Geometry check sheet. Reference: the model listing, model coordinates, mm. A direction names the side the tool comes from. Coordinates: 2 decimals unless noted, no trailing zeros. Write each loop counter-clockwise with the first axis right and the second up, starting at its lowest first coordinate (ties: lowest second). Pieces come first, ordered by that corner, then holes. Notation, with made-up numbers: (-27, -15) -> (28, -15) arc R27 ccw to (28, 12) -> close; hole circle Ø6 at (78, -32). An arc over 180 degrees is marked (long way). Answer in a Markdown table with one row per item. Add a question column.
1. Cross-section at D-D on z = -6.5. Record the cut outline in (x, y) (3 decimals), and give its area (3 significant figures).
2. Cross-section at C-C on x = 10. Record the cut outline in (y, z) (3 decimals).
3. Set-up check for faces 3 (the flat face through (0, -30, 3.35)), 4 (the flat face through (0, -61.675, 4)): record each of +Z, -Z, +X, -X, +Y, -Y from which the full face is reachable in a straight line by a thin tool's end or side.
4. Mould release check, pull along X, two halves, no side actions. Record for faces 1 (the cylindrical face through (-8.946, -31.269, -0.672)), 2 (the flat face through (0, 0, 4)): pulls with the +X half, pulls with the -X half, needs draft (parallel to the pull), parting line crosses it, or undercut.
5. Scan lines: L1, parallel to X at y = -46.5, z = -10; L2, parallel to Z at x = -1, y = -56.5; L3, parallel to Z at x = -9.5, y = -56. Record each from-to range of solid material in increasing order. Write a range as from..to.
6. Cross-section at B-B on y = -19. Record the cut outline in (x, z).
7. Depth check by flat-ended pin: P1, Ø5.5, axis at y = -43, z = -1.5, coming from the +X side; P2, Ø12, axis at y = -23, z = -12.5, coming from the -X side; P3, Ø1, axis at x = 6, y = -16.5, coming from the +Z side; P4, Ø3, axis at y = -16.5, z = -5, coming from the -X side. Enter the tip coordinate at first touch or a pass-through.
8. Cross-section at A-A on z = 10. Record the cut outline in (x, y) (3 decimals).
```python
from build123d import *

# Parameters (mm, degrees)
SKETCH1_W                   = 6.7
SKETCH1_H                   = 6.7
BOSS_EXTRUDE1_DEPTH         = 61.675
TAP_DRILL_FOR_M3X0_5_TAP1_D = 2.5


with BuildPart() as part:
    # Sketch1 → Boss-Extrude1 (new body)
    # profile 1 of 2: a face of its own
    with BuildSketch(Plane(origin=(0, 0, 0), x_dir=(1, 0, 0), z_dir=(0, 1, 0))):
        with BuildLine():
            ThreePointArc((0, -17.5), (12.374368671, -12.374368671), (17.5, 0))
            ThreePointArc((17.5, 0), (7.362522242, -7.362522242), (0, -17.5))
        make_face()
    # profile 2 of 2: a face of its own
    with BuildSketch(Plane(origin=(0, 0, 0), x_dir=(1, 0, 0), z_dir=(0, 1, 0))):
        with BuildLine():
            ThreePointArc((0, -17.5), (7.362522242, -7.362522242), (17.5, 0))
            ThreePointArc((17.5, 0), (-12.374368671, 12.374368671), (0, -17.5))
        make_face()
        Rectangle(SKETCH1_W, SKETCH1_H, mode=Mode.SUBTRACT)
    extrude(amount=-BOSS_EXTRUDE1_DEPTH)

    # Tap Drill for M3x0.5 Tap1 (through all)
    with Locations(Plane(origin=(0, 0, -10), x_dir=(0, 0, 1), z_dir=(0, 1, 0))):
        with Locations((0, 0), (10, 10), (10, -10), (20, 0)):
            Hole(TAP_DRILL_FOR_M3X0_5_TAP1_D / 2)


solid = part.part
```
Results found:
| question | item | result |
|---|---|---|
| 1 | outline | (-16.248, -61.675) -> (16.248, -61.675) -> (16.248, 0) -> (-16.248, 0) -> close |
| 1 | area | 2,000 mm^2 |
| 2 | outline | (-61.675, -14.361) -> (0, -14.361) -> (0, -1.25) -> (-61.675, -1.25) -> close; (-61.675, 1.25) -> (0, 1.25) -> (0, 14.361) -> (-61.675, 14.361) -> close |
| 3 | face 3 | +Y, -Y |
| 3 | face 4 | +Z, -Z, +X, -X, -Y |
| 4 | face 1 | undercut |
| 4 | face 2 | needs draft |
| 5 | L1 | x = -14.36..-1.25, 1.25..14.36 |
| 5 | L2 | z = -17.47..-10.75, -9.25..-3.35, 3.35..9.25, 10.75..17.47 |
| 5 | L3 | z = -14.7..-1.15, 1.15..14.7 |
| 6 | outline | circle Ø35 at (0, 0); hole circle Ø2.5 at (-10, 0); hole (-3.35, -3.35) -> (3.35, -3.35) -> (3.35, 3.35) -> (-3.35, 3.35) -> close; hole circle Ø2.5 at (0, -10); hole circle Ø2.5 at (0, 10); hole circle Ø2.5 at (10, 0) |
| 7 | P1 | stops at x = 17.5 |
| 7 | P2 | stops at x = -16.25 |
| 7 | P3 | stops at z = 16.61 |
| 7 | P4 | stops at x = -17.15 |
| 8 | outline | (-14.361, -61.675) -> (-1.25, -61.675) -> (-1.25, 0) -> (-14.361, 0) -> close; (1.25, -61.675) -> (14.361, -61.675) -> (14.361, 0) -> (1.25, 0) -> close |
